from build123d import *

# Parameters (mm, degrees)
F0_W     = 500
F0_H     = 410
F1_DEPTH = 410
F2_T     = -30
F3_W     = 500
F3_H     = 410
F4_DEPTH = 30


with BuildPart() as f1:
    # F0 (on Front) → F1 (new body)
    with BuildSketch(Plane.XZ):
        Rectangle(F0_W, F0_H)
    extrude(amount=-F1_DEPTH)

    # F2
    f2_openings = [f1.faces().sort_by_distance(p)[0] for p in [
        (0, 205, 205),
    ]]
    offset(amount=F2_T, openings=f2_openings)

    # F3 (on face) → F4 (join)
    with BuildSketch(Plane.XY.offset(205)):
        with Locations((0, 205)):
            Rectangle(F3_W, F3_H)
    extrude(amount=F4_DEPTH)


solid = f1.part
Model file for the job. Use its own axes, mm. A direction names the side the tool comes from. Give positions to 0.01 mm unless a question says otherwise; leave off trailing zeros. Loops run counter-clockwise (first coordinate to the right, second up) from the corner with the lowest first, then second, coordinate; pieces in that order, holes last.
1) Saw through at A-A (y = 338). Write the cut outline in (x, z), plus the area to 3 significant figures.
2) Wall check: line 1 (Z direction, x = 110.5, y = 86); line 2 (Y direction, x = 126, z = -87); line 3 (X direction, y = 332, z = -66). Give the ranges that are in metal, low to high.
3) Saw through at B-B (z = 46.5). Write the cut outline in (x, y), plus the area to 3 significant figures.
4) Tool access for faces 1 (the flat face through (-3, 30, 18)), 2 (the flat face through (250, 202, 12)): list every direction of +Z, -Z, +X, -X, +Y, -Y with a clear straight run to the whole face (end or side of a thin tool).
5) Pull direction X, two halves, no side cores. Call faces 3 (the flat face through (-250, 202, 12)), 4 (the flat face through (-3, 410, 12)), 5 (the flat face through (-3, 207, 205)), 6 (the flat face through (-3, 203, -175)): +X half, -X half, draft (parallel to the pull), parting line (faces both ways), or undercut.
Answer block:
1. outline: (-250, -205) - (250, -205) - (250, 235) - (-250, 235) - close; hole (-220, -175) - (220, -175) - (220, 205) - (-220, 205) - close
1. area: 52,800 mm2
2. line 1: z = -205 to -175, 205 to 235
2. line 2: y = 0 to 30, 380 to 410
2. line 3: x = -250 to -220, 220 to 250
3. outline: (-250, 0) - (250, 0) - (250, 410) - (-250, 410) - close; hole (-220, 30) - (220, 30) - (220, 380) - (-220, 380) - close
3. area: 51,000 mm2
4. face 1: none
4. face 2: +Z, -Z, +X, +Y, -Y
5. face 3: -X half
5. face 4: draft
5. face 5: undercut
5. face 6: undercut
